Could you check a few things on this drawing? It's one solid part, dimensions in mm from its lowest x, y, z. A direction names the side the tool comes from. Give positions to 0.01 mm unless a question says otherwise; leave off trailing zeros. Order: outer loops, then holes, each group sorted by start corner. A loop starts at its lowest first (then second) coordinate and runs counter-clockwise, first axis right, second up.
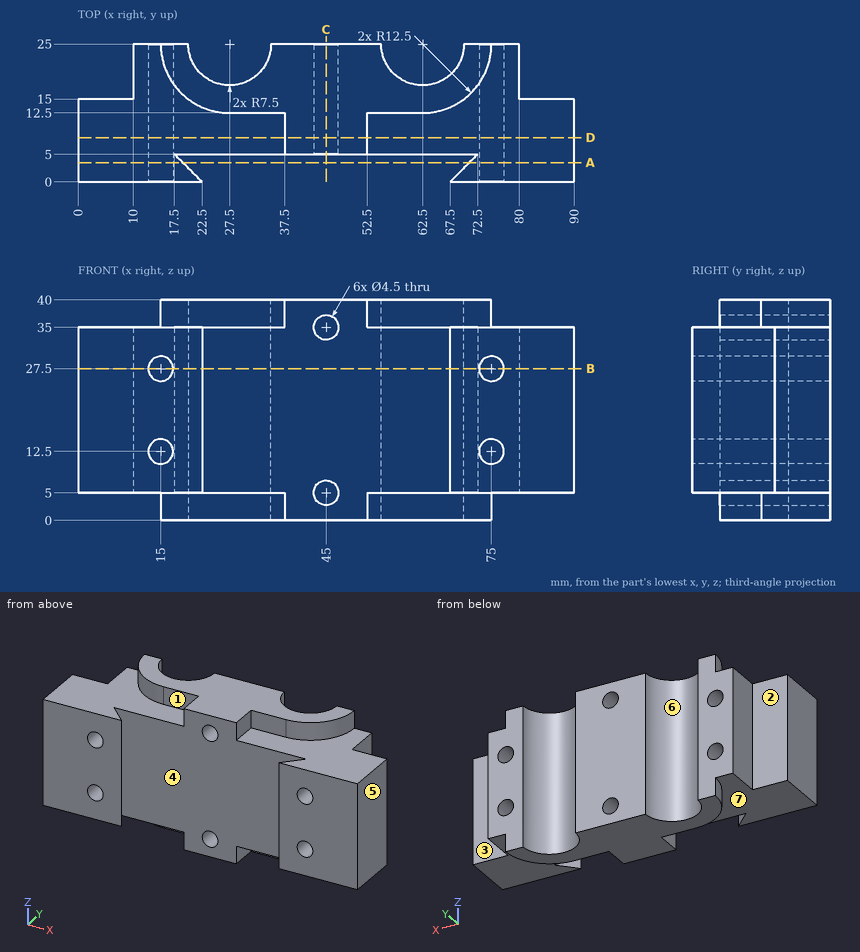
Q1. I need wall thicknesses on L1, parallel to Z at x = 45, y = 19.75; L2, parallel to Z at x = 75, y = 10; L3, parallel to X at y = 7, z = 27.5. Which ranges of each line are inside material? Lowest first, please.
Filled sheet:
L1: z = 0 to 2.75, 7.25 to 32.75, 37.25 to 40
L2: z = 5 to 10.25, 14.75 to 25.25, 29.75 to 35
L3: x = 0 to 12.75, 17.25 to 72.75, 77.25 to 90
Q2. If we section it at C-C on x = 45: List the corners of the cut face in (y, z) for me.
Filled sheet:
outline: (5, 0) - (25, 0) - (25, 2.75) - (5, 2.75) - close; (5, 7.25) - (25, 7.25) - (25, 32.75) - (5, 32.75) - close; (5, 37.25) - (25, 37.25) - (25, 40) - (5, 40) - close
Q3. For the marked faces 1, 2, 3 and 4, which set-ups out of +Z, -Z, +X, -X, +Y, -Y let a thin tool reach every point of the face, with its end or its side?
Filled sheet:
face 1: +Z, -X, -Y
face 2: +Z, -Z, -X, +Y
face 3: +Z, -Z, +X, +Y
face 4: +Z, -Z
Q4. If we section it at B-B on z = 27.5: List the corners of the cut face in (x, y) for me, plus the area to 3 significant figures.
Filled sheet:
outline: (0, 0) - (12.75, 0) - (12.75, 25) - (10, 25) - (10, 15) - (0, 15) - close; (17.25, 0) - (22.5, 0) - (17.5, 5) - (72.5, 5) - (67.5, 0) - (72.75, 0) - (72.75, 25) - (70, 25) arc R7.5 cw to (55, 25) - (35, 25) arc R7.5 cw to (20, 25) - (17.25, 25) - close; (77.25, 0) - (90, 0) - (90, 15) - (80, 15) - (80, 25) - (77.25, 25) - close
area: 1,400 mm2
Q5. I'm going to push flat-ended pins straight in: P1, Ø1.5, axis at x = 60, z = 37, coming from the -Y side; P2, Ø1, axis at y = 20, z = 10.5, coming from the -X side; P3, Ø1, axis at x = 61, y = 3, coming from the +Z side; P4, Ø11, axis at x = 4, z = 24, coming from the +Y side. Where does each tip first touch, or does it pass through?
Filled sheet:
P1: stops at y = 12.5
P2: stops at x = 10
P3: passes through
P4: stops at y = 15
Q6. If we section it at A-A on y = 3.5: List the corners of the cut face in (x, z) for me.
Filled sheet:
outline: (0, 5) - (19, 5) - (19, 35) - (0, 35) - close; (71, 5) - (90, 5) - (90, 35) - (71, 35) - close; hole circle Ø4.5 at (15, 12.5); hole circle Ø4.5 at (15, 27.5); hole circle Ø4.5 at (75, 12.5); hole circle Ø4.5 at (75, 27.5)
Q7. If we section it at D-D on y = 8: List the corners of the cut face in (x, z) for me.
Filled sheet:
outline: (0, 5) - (37.5, 5) - (37.5, 0) - (52.5, 0) - (52.5, 5) - (90, 5) - (90, 35) - (52.5, 35) - (52.5, 40) - (37.5, 40) - (37.5, 35) - (0, 35) - close; hole circle Ø4.5 at (15, 12.5); hole circle Ø4.5 at (15, 27.5); hole circle Ø4.5 at (45, 5); hole circle Ø4.5 at (45, 35); hole circle Ø4.5 at (75, 12.5); hole circle Ø4.5 at (75, 27.5)
Q8. Thinking about a two-plate mould opening in X: for the marked faces 5, 6 and 7, which applies, released by +X, released by -X, zero draft, split by the parting line, or undercut?
Filled sheet:
face 5: released by +X
face 6: undercut
face 7: zero draft
